from build123d import *

# Parameters (mm, degrees)
F0_W           = 28
F0_H           = 19
F0_W_2         = 6
F1_DEPTH       = 5
F2_DEPTH       = 30
F3_R           = 14.99999
F6_D           = 4
F6_CBORE_D     = 8.5
F6_CBORE_DEPTH = 2.5
F7_R           = 2
F8_DEPTH       = 3
F10_DEPTH      = 214.001


# Not quite as in the source:
# - a fillet or chamfer is up to 0.001 mm smaller than in the source, because OpenCascade refuses the exact size
# - a feature names something its author has since deleted; it is built from what else it names


with BuildPart() as f1:
    # F0 (on Top) → F1 (new body)
    with BuildSketch(Plane.XY):
        Polygon((-107, 13.5), (-107, -13.5), (-51, -13.5), (-51, -9.5), (-65, -9.5), (-71, -9.5), (-99, -9.5), (-99, 9.5), (-71, 9.5), (-65, 9.5), (-51, 9.5), (-51, 13.5), align=None)
        Polygon((-51, -9.5), (-51, -13.5), (51, -13.5), (51, -9.5), (37, -9.5), (37, 9.5), (51, 9.5), (51, 13.5), (-51, 13.5), (-51, 9.5), (-37, 9.5), (-37, -9.5), align=None)
        with Locations((-17, 0)):
            Rectangle(F0_W, F0_H, mode=Mode.SUBTRACT)
        with Locations((17, 0)):
            Rectangle(F0_W, F0_H, mode=Mode.SUBTRACT)
        Polygon((51, -9.5), (51, -13.5), (107, -13.5), (107, 13.5), (51, 13.5), (51, 9.5), (65, 9.5), (71, 9.5), (99, 9.5), (99, -9.5), (71, -9.5), (65, -9.5), align=None)
        with Locations((-68, 0)):
            Rectangle(F0_W_2, F0_H)
        with Locations((68, 0)):
            Rectangle(F0_W_2, F0_H)
    extrude(amount=-F1_DEPTH)

    # F0 (on Top) → F2 (join)
    with BuildSketch(Plane.XY):
        Polygon((51, -9.5), (51, -13.5), (107, -13.5), (107, 13.5), (51, 13.5), (51, 9.5), (65, 9.5), (71, 9.5), (99, 9.5), (99, -9.5), (71, -9.5), (65, -9.5), align=None)
        Polygon((-107, 13.5), (-107, -13.5), (-51, -13.5), (-51, -9.5), (-65, -9.5), (-71, -9.5), (-99, -9.5), (-99, 9.5), (-71, 9.5), (-65, 9.5), (-51, 9.5), (-51, 13.5), align=None)
    extrude(amount=F2_DEPTH)

    # F3 (radius 15 in the source; OpenCascade refuses exactly that, so slightly less here)
    f3_edges = [f1.edges().sort_by_distance(p)[0] for p in [
        (51, 11.5, 0),
        (51, 11.5, 30),
        (-51, 11.5, 30),
        (-51, 11.5, 0),
        (-51, -11.5, 30),
        (51, -11.5, 30),
    ]]
    fillet(f3_edges, radius=F3_R)

    # F6 (through all)
    with Locations(Plane.XZ.offset(13.5)):
        with Locations((-79, 22), (79, 22), (-64, 22), (64, 22)):
            CounterBoreHole(F6_D / 2, F6_CBORE_D / 2, F6_CBORE_DEPTH)

    # F7 (on face) → F8 (cut)
    with BuildSketch(Plane(origin=(0, 13.5, 0), x_dir=(-1, 0, 0), z_dir=(0, 1, 0))):
        Polygon((-81.1656275844, 18.1837989441), (-76.7778867319, 18.2164109688), (-74.6122591474, 22.0326120247), (-76.8343724156, 25.8162010559), (-81.2221132681, 25.7835890312), (-83.3877408526, 21.9673879753), align=None)
        with Locations((-79, 22)):
            Circle(F7_R, mode=Mode.SUBTRACT)
        Polygon((-59.6121379542, 22), (-61.8060689771, 25.8), (-66.1939310229, 25.8), (-68.3878620458, 22), (-66.1939310229, 18.2), (-61.8060689771, 18.2), align=None)
        with Locations((-64, 22)):
            Circle(F7_R, mode=Mode.SUBTRACT)
        Polygon((61.8060689771, 18.2), (66.1939310229, 18.2), (68.3878620458, 22), (66.1939310229, 25.8), (61.8060689771, 25.8), (59.6121379542, 22), align=None)
        with Locations((64, 22)):
            Circle(F7_R, mode=Mode.SUBTRACT)
        Polygon((76.7778867319, 18.2164109688), (81.1656275844, 18.1837989441), (83.3877408526, 21.9673879753), (81.2221132681, 25.7835890312), (76.8343724156, 25.8162010559), (74.6122591474, 22.0326120247), align=None)
        with Locations((79, 22)):
            Circle(F7_R, mode=Mode.SUBTRACT)
    extrude(amount=-F8_DEPTH, mode=Mode.SUBTRACT)

    # F9 (on face) → F10 (cut, through all)
    with BuildSketch(Plane(origin=(-107, 0, 0), x_dir=(0, -1, 0), z_dir=(-1, 0, 0))):
        Polygon((-4.75, 6), (4.75, 6), (9.5, 14.227241336), (4.75, 22.4544826719), (-4.75, 22.4544826719), (-9.5, 14.227241336), align=None)
    extrude(amount=-F10_DEPTH, mode=Mode.SUBTRACT)


solid = f1.part
Model file for the job. Use its own axes, mm. A direction names the side the tool comes from. Give positions to 0.01 mm unless a question says otherwise; leave off trailing zeros. Loops run counter-clockwise (first coordinate to the right, second up) from the corner with the lowest first, then second, coordinate; pieces in that order, holes last. Notation, with made-up numbers: (-31, 19.5) -> (-18, 19.5) arc R15 cw to (-18, 44.5) -> close; hole circle Ø7 at (46, 88). An arc over 180 degrees is marked (long way). Use a Markdown table: item, result. Add a question column.
(1) Slice it at C-C on x = -43. List the corners of the cut face in (y, z), and give its area (3 significant figures).
(2) Drop flat-ended pins along their axis: pin 1 Ø1.5 at (y, z) = (4.5, 6.5) entering from -X; pin 2 Ø6 at (x, y) = (-25, 7) entering from +Z; pin 3 Ø5 at (x, z) = (-64, 22) entering from +Y. Give the stop position or say it passes through.
(3) Slice it at A-A on x = -79. List the corners of the cut face in (y, z).
(4) Wall check: line 1 along X through (y, z) = (-8.25, 3); line 2 along Y through (x, z) = (-80, -3); line 3 along Y through (x, z) = (-64.5, 19.5). Give the ranges that are in metal, low to high.
(5) Mould opens along Z. For faces 4 (the cylindrical face through (36.49, 0.94, 0.01)), 5 (the cylindrical face through (-80.908, 10.007, 22.601)), 6 (the flat face through (74, 9.5, 13)) say: +Z half, -Z half, draft (parallel to the pull), parting line (faces both ways), or undercut.
(6) Slice it at D-D on y = 1. Give the number of separate pieces and of enclosed holes in the cut face, and give its area (3 significant figures).
(7) Slice it at B-B on z = 10. List the corners of the cut face in (x, y).
(8) Tool access for faces 1 (the flat face through (-1, 0, 0)), 2 (the flat face through (-71, 0, -2)), 3 (the flat face through (-68, 0, 0)): list every direction of +Z, -Z, +X, -X, +Y, -Y with a clear straight run to the whole face (end or side of a thin tool).
Filled sheet:
| question | item | result |
|---|---|---|
| 1 | outline | (-13.5, -5) -> (-9.5, -5) -> (-9.5, 1.73) -> (-13.5, 1.73) -> close; (9.5, -5) -> (13.5, -5) -> (13.5, 1.73) -> (9.5, 1.73) -> close |
| 1 | area | 53.9 mm2 |
| 2 | pin 1 | x = -107 |
| 2 | pin 2 | z = 0 |
| 2 | pin 3 | y = 10.5 |
| 3 | outline | (-13.5, -5) -> (-9.5, -5) -> (-9.5, 20) -> (-11, 20) -> (-11, 17.75) -> (-13.5, 17.75) -> close; (-13.5, 26.25) -> (-11, 26.25) -> (-11, 24) -> (-9.5, 24) -> (-9.5, 30) -> (-13.5, 30) -> close; (9.5, -5) -> (13.5, -5) -> (13.5, 18.2) -> (10.5, 18.2) -> (10.5, 20) -> (9.5, 20) -> close; (9.5, 24) -> (10.5, 24) -> (10.5, 25.8) -> (13.5, 25.8) -> (13.5, 30) -> (9.5, 30) -> close |
| 4 | line 1 | -107 to -99, 99 to 107 |
| 4 | line 2 | -13.5 to -9.5, 9.5 to 13.5 |
| 4 | line 3 | -11 to -9.5, 9.5 to 10.5 |
| 5 | face 4 | +Z half |
| 5 | face 5 | undercut |
| 5 | face 6 | draft |
| 6 | separate pieces | 9 |
| 6 | enclosed holes | 0 |
| 6 | area | 447 mm2 |
| 7 | outline | (-107, -13.5) -> (-50.14, -13.5) -> (-50.14, -9.5) -> (-99, -9.5) -> (-99, -7.06) -> (-107, -7.06) -> close; (-107, 7.06) -> (-99, 7.06) -> (-99, 9.5) -> (-50.14, 9.5) -> (-50.14, 13.5) -> (-107, 13.5) -> close; (50.14, -13.5) -> (107, -13.5) -> (107, -7.06) -> (99, -7.06) -> (99, -9.5) -> (50.14, -9.5) -> close; (50.14, 9.5) -> (99, 9.5) -> (99, 7.06) -> (107, 7.06) -> (107, 13.5) -> (50.14, 13.5) -> close |
| 8 | face 1 | +Z, +Y, -Y |
| 8 | face 2 | +Z, -Z |
| 8 | face 3 | +Z |
